Solid Edge part; units mm, degrees
sketch "Sketch1" plane through (0, 0, 0) normal (0, 0, 1) x (1, 0, 0)
  line L0 (-32.5, -20) -> (32.5, -20)
  line L1 (32.5, -20) -> (32.5, 20)
  line L2 (32.5, 20) -> (-32.5, 20)
  line L3 (-32.5, 20) -> (-32.5, -20)
extrude "Protrusion1" add sketch "Sketch1" against normal blind 40
sketch "Sketch2" plane through (0, 0, 0) normal (0, 0, 1) x (1, 0, 0)
  line L0 (-32.5, -2.75) -> (32.5, -2.75)
  line L1 (32.5, -2.75) -> (32.5, 2.75)
  line L2 (32.5, 2.75) -> (-32.5, 2.75)
  line L3 (-32.5, 2.75) -> (-32.5, -2.75)
extrude "ExtrudedCutout_1" cut sketch "Sketch2" against normal blind 28
fillet "Round_1" radius 2 1 edges at (0, 20, -40)
chamfer "Chamfer_6" distance 12 angle 30 1 edges at (32.5, 2.75, -14) measured on face at (22.3167, 2.75, -23.0533)
chamfer "Chamfer_7" distance 12 angle 30 1 edges at (32.5, 3.4641, -28) measured on face at (-22.3167, -0.5544, -28)
chamfer "Chamfer_8" distance 12 angle 30 1 edges at (32.5, -2.75, -17.4641) measured on face at (-22.3167, -2.75, -17.1148)
chamfer "Chamfer_9" distance 12 angle 30 1 edges at (-32.5, -2.75, -14) measured on face at (-24.1967, -2.75, -23.0533)
chamfer "Chamfer_10" distance 12 angle 30 1 edges at (-32.5, 2.75, -14) measured on face at (12.1967, 2.75, -23.0533)
chamfer "Chamfer_11" distance 12 angle 30 1 edges at (-32.5, 0, -28) measured on face at (-24.1967, 0.1936, -28)
Read the model definition and answer for the solid it produces. Units are mm, in the model's axes. A direction names the side the tool comes from. Round coordinates to 2 decimals unless told otherwise and drop trailing zeros. Write each loop counter-clockwise with the first axis right and the second up, starting at its lowest first coordinate (ties: lowest second). Pieces come first, ordered by that corner, then holes. Notation, with made-up numbers: M 59,61.25 L 75,61.25 A16 ccw 75,78.25 Z; hole C 69.5,84.25 d11. An arc over 180 degrees is marked long. Use a Markdown table: item, result.
1) Flat-ended cylindrical pins translate along their axes: pin 1 (3 mm diameter, centred on x = 9.5, y = 0, fed in from +Z); pin 2 (12 mm diameter, centred on y = -7.5, z = -27.5, fed in from -X). Find the tip coordinate at first contact, or state that the pin passes through.
Answers follow:
| item | result |
|---|---|
| pin 1 | stops at z = -28 |
| pin 2 | stops at x = -32.5 |
2) The part is cut by section A-A (z = -16). Write down the section's boundary in (x, y).
Answers follow:
| item | result |
|---|---|
| outline | M -32.5,-20 L 32.5,-20 L 32.5,-9.68 L 20.5,-2.75 L -20.5,-2.75 L -32.5,-9.68 Z; M -32.5,9.68 L -20.5,2.75 L 20.5,2.75 L 32.5,9.68 L 32.5,20 L -32.5,20 Z |
3) Straight lines are drawn through the part: line 1 along Y through (x, z) = (-0.5, -17); line 2 along Y through (x, z) = (24, -7); line 3 along Z through (x, y) = (18, 0). For each, find the intervals that lie inside material, in ascending order. Write a range as [from, to].
Answers follow:
| item | result |
|---|---|
| line 1 | y = [-20, -2.75], [2.75, 20] |
| line 2 | y = [-20, -4.77], [4.77, 20] |
| line 3 | z = [-40, -28] |
4) A tool of negligible diameter and unlimited length cuts with its end or side. For faces 1 (the flat face through (-27.917, -0.135, -32.282)), 2 (the flat face through (0, 2.75, -14)), 3 (the flat face through (26.58, 6.26, -17.71)), from which of +Z, -Z, +X, -X, +Y, -Y can it reach the whole face along a straight path? Write none if from no direction.
Answers follow:
| item | result |
|---|---|
| face 1 | +Z, -X |
| face 2 | +Z, +X, -X |
| face 3 | +Z, +X |
5) The part is cut by section C-C (y = -8.5). Write down the section's boundary in (x, z).
Answers follow:
| item | result |
|---|---|
| outline | M -32.5,-40 L 32.5,-40 L 32.5,-34.93 L 30.46,-33.75 L 30.46,0 L -30.46,0 L -30.46,-33.75 L -32.5,-34.93 Z |
6) The part is cut by section D-D (z = -32). Write down the section's boundary in (x, y).
Answers follow:
| item | result |
|---|---|
| outline | M -32.5,-20 L 32.5,-20 L 32.5,-9.68 L 27.43,-6.75 L 27.43,6.75 L 32.5,9.68 L 32.5,20 L -32.5,20 L -32.5,9.68 L -27.43,6.75 L -27.43,-6.75 L -32.5,-9.68 Z |
7) The part is cut by section B-B (x = -4.5). Write down the section's boundary in (y, z).
Answers follow:
| item | result |
|---|---|
| outline | M -20,-40 L 18,-40 A2 ccw 20,-38 L 20,0 L 2.75,0 L 2.75,-28 L -2.75,-28 L -2.75,0 L -20,0 Z |
